The listing builds one solid part. Answer for the finished solid, in the listing's coordinates (mm). Round coordinates to 2 decimals unless told otherwise and drop trailing zeros. Write each loop counter-clockwise with the first axis right and the second up, starting at its lowest first coordinate (ties: lowest second). Pieces come first, ordered by that corner, then holes. Notation, with made-up numbers: (18.25, -15) - (51.25, -15) arc R13 ccw to (51.25, 8) - close; hole circle Ø2 at (-5.75, 44). An arc over 180 degrees is marked (long way). Return JSON: item names as keys, results as strings. Group by question number.
(1) Find the intervals of material crossed by line 1 along X through (y, z) = (-5.75, 44.45); line 2 along X through (y, z) = (-16.75, 38); line 3 along X through (y, z) = (-8.75, 83), in increasing order. Write a range as [from, to].
(2) Section A-A, the plane y = -15.25 is taken. Write down the section's boundary in (x, z) (3 decimals), then the cut area to 3 significant figures.
(3) Section B-B, the plane z = 16 is taken. Write down the section's boundary in (x, y), then the cut area to 3 significant figures.
(4) Determine the mould class of faces 1 (the cylindrical face through (-419.11, -9.66, 45.44)), 2 (the cylindrical face through (-19.06, -9.66, 44.03)), 3 (the flat face through (-412, -9, 0)), 4 (the flat face through (-442, -9, 88.9)) for opening direction Z: +Z half, -Z half, draft (parallel to the pull), parting line (faces both ways), or undercut.
(5) Each of these flat-tipped pins is pushed along its axis until it touches: pin 1 (1.5 mm diameter, centred on x = -457.5, z = 27.5, fed in from +Y); pin 2 (3 mm diameter, centred on y = -2.5, z = 12, fed in from -X); pin 3 (6 mm diameter, centred on y = -3, z = 18.5, fed in from -X); pin 4 (11.5 mm diameter, centred on x = -28.575, z = 44.45, fed in from +Y). Where does it stop, or does it pass through?
```python
from build123d import *

# Parameters (mm, degrees)
F1_DEPTH = 19.05
F3_D     = 19.05
F5_D     = 19.05


with BuildPart() as f1:
    # F0 (on Front) → F1 (new body)
    with BuildSketch(Plane.XZ):
        Polygon((-812.273561069, 0), (0, 0), (0, 31.75), (-32.9955678842, 88.9), (-863.6, 88.9), align=None)
    extrude(amount=F1_DEPTH)

    # F3 (through all)
    with Locations(Plane(origin=(0, 0, 0), x_dir=(1, 0, 0), z_dir=(0, 1, 0))):
        with Locations((-28.575, -44.45)):
            Hole(F3_D / 2)

    # F5 (through all)
    with Locations(Plane(origin=(0, 0, 0), x_dir=(1, 0, 0), z_dir=(0, 1, 0))):
        with Locations((-428.625, -45.8583533764)):
            Hole(F5_D / 2)


solid = f1.part
```
Working result:
{
 "1": {"line 1": "x = [-837.94, -438.05], [-419.2, -38.1], [-19.05, -7.33]", "line 2": "x = [-834.21, -434.01], [-423.24, -35.58], [-21.57, -3.61]", "line 3": "x = [-860.19, -29.59]"},
 "2": {"outline": "(-863.6, 88.9) - (-812.274, 0) - (0, 0) - (0, 31.75) - (-32.996, 88.9) - close; hole circle Ø19.05 at (-428.625, 45.858); hole circle Ø19.05 at (-28.575, 44.45)", "area": "73,000 mm^2"},
 "3": {"outline": "(-821.51, -19.05) - (0, -19.05) - (0, 0) - (-821.51, 0) - close", "area": "15,600 mm^2"},
 "4": {"face 1": "undercut", "face 2": "undercut", "face 3": "-Z half", "face 4": "+Z half"},
 "5": {"pin 1": "stops at y = 0", "pin 2": "stops at x = -820.07", "pin 3": "stops at x = -824.69", "pin 4": "passes through"}
}
